```python
from build123d import *

# Parameters (mm, degrees)
F0_R     = 50.8
F1_DEPTH = 25.4
F2_R     = 7.62
F3_T     = -2.54


# Not quite as in the source:
# - a shell that OpenCascade refuses in one call is made with other operations: the cavity is built on its own and cut out


with BuildPart() as f1:
    # F0 (on Front) → F1 (new body)
    with BuildSketch(Plane.XZ):
        Circle(F0_R)
    extrude(amount=F1_DEPTH)

    # F2
    f2_edges = [f1.edges().sort_by_distance(p)[0] for p in [
        (-50.8, -25.4, 0),
        (-50.8, 0, 0),
    ]]
    fillet(f2_edges, radius=F2_R)

    # F3: a shell. OpenCascade refuses it in one call, so the cavity is built on its own and cut out:
    # the body offset inwards by the wall thickness, plus a prism from it out through each open face.
    f3_core = offset(f1.part, amount=F3_T, mode=Mode.PRIVATE)
    f3_exits = [f3_core.faces().sort_by_distance(p)[0] for p in [
        (0, -22.86, 0),
        (0, -2.54, 0),
    ]]
    add(f3_core, mode=Mode.SUBTRACT)
    extrude(f3_exits, amount=-F3_T, mode=Mode.SUBTRACT)


solid = f1.part
```
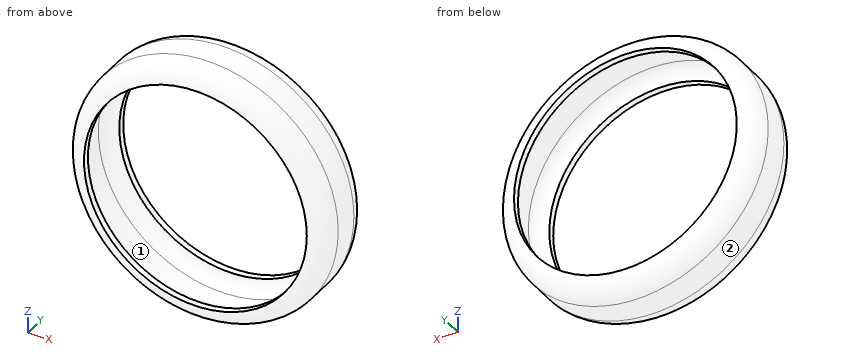
Source: CAD feature listing. Evaluate the final solid. Frame: model axes, mm. Face numbers are marked on the shaded views. Coordinates: 2 decimals unless noted, no trailing zeros. Loops run counter-clockwise (first coordinate to the right, second up) from the corner with the lowest first, then second, coordinate; pieces in that order, holes last. Notation, with made-up numbers: M 34.5,-27.5 L 59.5,-27.5 A17 cw 59.5,-19.5 Z; hole C -34,-13 d6. An arc over 180 degrees is marked long. Put each result on its own line as item: value. Start each with the question number.
1) Cut plane C-C on y = -15.75. Return the cut outline in (x, z), then the cut area to 3 significant figures.
2) Contact query for flat-ended pins moving along their axis: pin 1 Ø3 at (y, z) = (-16, 17.5) entering from +X; pin 2 Ø4 at (y, z) = (-5.5, -20) entering from -X; pin 3 Ø1.5 at (x, y) = (18.5, -21) entering from -Z. Output: stop coordinate, or through.
3) Ray query, L1, parallel to Z at x = 0, y = -13.25; L2, parallel to Z at x = -26, y = -17; L3, parallel to X at y = -23.75, z = -39.5. Return the intervals inside material, ascending. Write a range as from..to.
4) Cut plane B-B on x = 0. Return the cut outline in (y, z).
5) Cut plane A-A on z = 0. Return the cut outline in (x, y), then the cut area to 3 significant figures.
6) Pull-direction query (Z, two-part tool) for the marked faces 1 and 2; classes: pulls with the +Z half, pulls with the -Z half, needs draft (parallel to the pull), parting line crosses it, or undercut.
7) Cut plane D-D on y = -4.25. Return the cut outline in (x, z), then the cut area to 3 significant figures.
The answers:
1. outline: C 0,0 d101.6; hole C 0,0 d96.52
1. area: 790 mm²
2. pin 1: stops at x = 48.21
2. pin 2: stops at x = -47.32
2. pin 3: stops at z = -46.99
3. L1: z = -50.8..-48.26, 48.26..50.8
3. L2: z = -43.64..-40.66, 40.66..43.64
3. L3: x = -27.12..-17.44, 17.44..27.12
4. outline: M -25.4,-43.18 A7.62 ccw -17.78,-50.8 L -7.62,-50.8 A7.62 ccw 0,-43.18 L -2.54,-43.18 A5.08 cw -7.62,-48.26 L -17.78,-48.26 A5.08 cw -22.86,-43.18 Z; M -25.4,43.18 L -22.86,43.18 A5.08 cw -17.78,48.26 L -7.62,48.26 A5.08 cw -2.54,43.18 L 0,43.18 A7.62 ccw -7.62,50.8 L -17.78,50.8 A7.62 ccw Z
5. outline: M -50.8,-17.78 A7.62 ccw -43.18,-25.4 L -43.18,-22.86 A5.08 cw -48.26,-17.78 L -48.26,-7.62 A5.08 cw -43.18,-2.54 L -43.18,0 A7.62 ccw -50.8,-7.62 Z; M 43.18,-25.4 A7.62 ccw 50.8,-17.78 L 50.8,-7.62 A7.62 ccw 43.18,0 L 43.18,-2.54 A5.08 cw 48.26,-7.62 L 48.26,-17.78 A5.08 cw 43.18,-22.86 Z
5. area: 153 mm²
6. face 1: undercut
6. face 2: parting line crosses it
7. outline: C 0,0 d100.03; hole C 0,0 d93.96
7. area: 924 mm²
